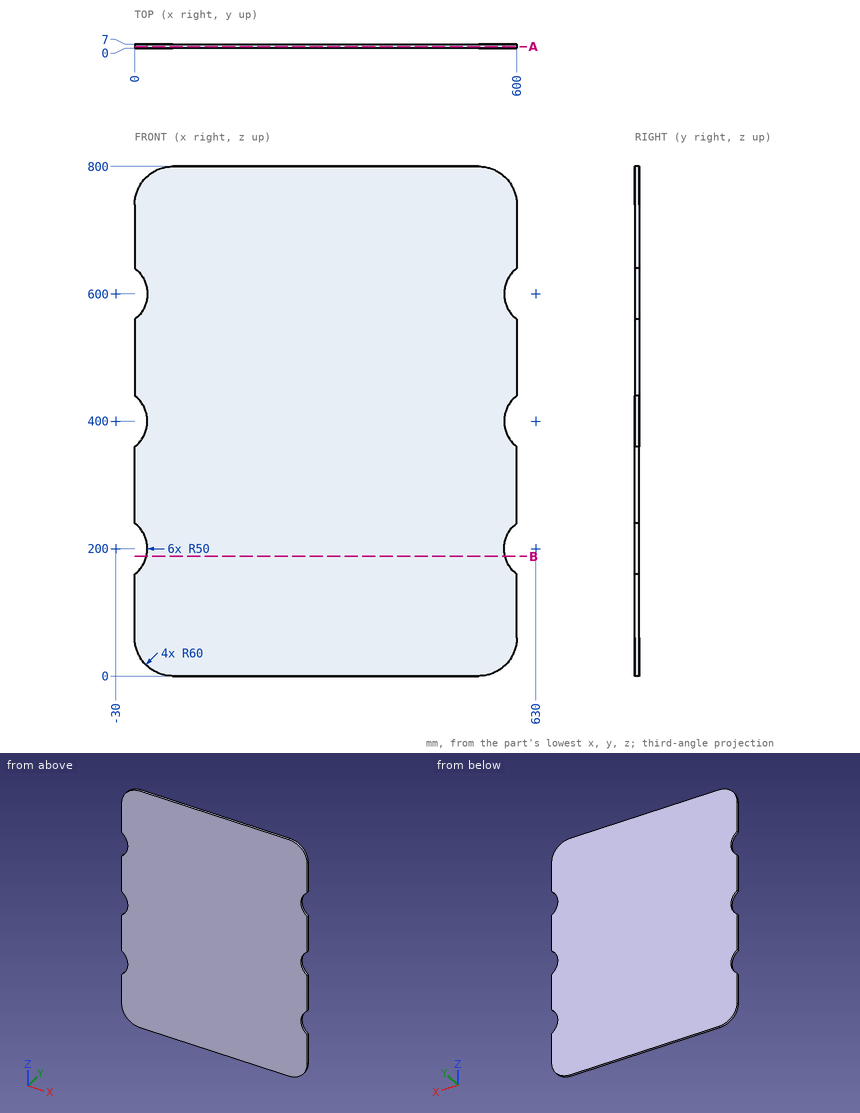
The drawing under review shows one solid part. Ordinate dimensions are in mm from its lowest x, y, z. Round coordinates to 2 decimals unless told otherwise and drop trailing zeros. Write each loop counter-clockwise with the first axis right and the second up, starting at its lowest first coordinate (ties: lowest second). Pieces come first, ordered by that corner, then holes. Notation, with made-up numbers: (65.25, 47.5) - (74.25, 47.5) arc R24 ccw to (74.25, 76.5) - close; hole circle Ø7 at (56, 58.5). An arc over 180 degrees is marked (long way). Put each result on its own line as item: value.
Q1. We need section B-B (z = 188). Give the boundary of the cut face in (x, y).
Solved:
outline: (18.54, 0) - (581.46, 0) - (581.46, 7) - (18.54, 7) - close
Q2. Wall thickness on probe 1 along X at (y, z) = (4, 56.5); probe 2 along Z at (x, y) = (561, 1.25); probe 3 along X at (y, z) = (2.5, 421): over which ranges is each line inside the solid? List them lowest first.
Solved:
probe 1: x = 0.1 to 599.9
probe 2: z = 3.8 to 796.2
probe 3: x = 15.38 to 584.62
Q3. We need section A-A (y = 3). Give the boundary of the cut face in (x, z), and give its area (3 significant figures).
Solved:
outline: (0, 60) arc R60 ccw to (60, 0) - (540, 0) arc R60 ccw to (600, 60) - (600, 160) arc R50 cw to (600, 240) - (600, 360) arc R50 cw to (600, 440) - (600, 560) arc R50 cw to (600, 640) - (600, 740) arc R60 ccw to (540, 800) - (60, 800) arc R60 ccw to (0, 740) - (0, 640) arc R50 cw to (0, 560) - (0, 440) arc R50 cw to (0, 360) - (0, 240) arc R50 cw to (0, 160) - close
area: 470,000 mm2
Q4. Insertion check: pin 1 Ø1 at (y, z) = (4, 409.5) entering from +X. The pin has a flat end and moves straight along its axis. Give the tip position at first contact, or say it passes through.
Solved:
pin 1: stops at x = 581.01
